from build123d import *

# Parameters (mm, degrees)
EXTRUDE1_DEPTH        = 3
SKETCH2_R             = 4
EXTRUDE2_DEPTH        = 9.5
SKETCH3_R             = 3
EXTRUDE3_DEPTH        = 11.5
SKETCH4_R             = 1.25
EXTRUDE4_DEPTH        = 10
SKETCH5_R             = 1.5
EXTRUDE5_DEPTH        = 3
M3_TAPPED_HOLE1_D     = 2.5
M3_TAPPED_HOLE1_DEPTH = 7.5
M3_TAPPED_HOLE1_TIP   = 0.751075774


with BuildPart() as part:
    # Sketch1 → Extrude1 (new body)
    with BuildSketch(Plane.XY):
        with BuildLine():
            Line((10, 4), (0, 4))
            ThreePointArc((0, 4), (-2.828427125, 2.828427125), (-4, 0))
            Line((-4, 0), (-4, -10))
            ThreePointArc((-4, -10), (5.899494937, -5.899494937), (10, 4))
        make_face()
    extrude(amount=EXTRUDE1_DEPTH)

    # Sketch2 → Extrude2 (add)
    with BuildSketch(Plane.XY.offset(3)):
        with Locations(Location((0, 0, 0), (0, 0, 180))):
            Circle(SKETCH2_R)
    extrude(amount=EXTRUDE2_DEPTH)

    # Sketch3 → Extrude3 (add)
    with BuildSketch(Plane.XY.offset(12.5)):
        Circle(SKETCH3_R)
    extrude(amount=EXTRUDE3_DEPTH)

    # Sketch4 → Extrude4 (cut)
    with BuildSketch(Plane.XY.offset(24)):
        Circle(SKETCH4_R)
    extrude(amount=-EXTRUDE4_DEPTH, mode=Mode.SUBTRACT)

    # Sketch5 → Extrude5 (cut)
    with BuildSketch(Plane.XY.offset(3)):
        with Locations((7, 1)):
            Circle(SKETCH5_R)
        with Locations((-1, -7)):
            Circle(SKETCH5_R)
    extrude(amount=-EXTRUDE5_DEPTH, mode=Mode.SUBTRACT)

    # M3 Tapped Hole1
    with Locations(Plane.XY.offset(24)):
        with Locations((0, 0)):
            Hole(M3_TAPPED_HOLE1_D / 2, depth=M3_TAPPED_HOLE1_DEPTH)
            with Locations((0, 0, -(M3_TAPPED_HOLE1_DEPTH + M3_TAPPED_HOLE1_TIP / 2))):  # 118° drill point
                Cone(0, M3_TAPPED_HOLE1_D / 2, M3_TAPPED_HOLE1_TIP, mode=Mode.SUBTRACT)


solid = part.part
Verification items for the finished model (mm, model axes). A direction names the side the tool comes from. Give positions to 0.01 mm unless a question says otherwise; leave off trailing zeros. Loops run counter-clockwise (first coordinate to the right, second up) from the corner with the lowest first, then second, coordinate; pieces in that order, holes last. Notation, with made-up numbers: (77.25, 28) - (114.25, 28) arc R37 cw to (114.25, 64) - close; hole circle Ø1 at (-39, 35.5). An arc over 180 degrees is marked (long way). Write item = value, one per line. Start each with the question number.
Q1. Mould release check, pull along Y, two halves, no side actions. Record for faces 3 (the face through (-0.27, -1.22, 19.07)), 4 (the face through (-1, -3, 12.5)), 5 (the face through (-1.325, -8.464, 1.521)), 6 (the face through (-3, 0, 18)): released by +Y, released by -Y, zero draft, split by the parting line, or undercut.
Q2. Depth check by flat-ended pin: P1, Ø5, axis at y = -5, z = 7.5, coming from the +X side; P2, Ø3, axis at y = 2, z = 10.5, coming from the -X side; P3, Ø3, axis at x = 5, y = 1.5, coming from the +Z side; P4, Ø2, axis at y = -4.5, z = 20.5, coming from the -X side. Enter the tip coordinate at first touch or a pass-through.
Q3. Tool access check on faces 1 (the face through (5.5, 1.07, 1.52)), 2 (the face through (0, 0, 14)). Record the directions out of +Z, -Z, +X, -X, +Y, -Y that give a thin tool (end or side, any length) a straight path to the whole face; none if there is none.
Q4. Cross-section at A-A, the plane y = 1. Enter the section's corners in (x, z).
Q5. Thickness scan on line 1 (Y direction, x = 0, z = 18.5); line 2 (Y direction, x = 7, z = 2.1); line 3 (Z direction, x = 1.5, y = -7.25). Record the ranges inside material, lowest first.
Q6. Cross-section at B-B, the plane x = -1. Enter the section's corners in (y, z).
Q7. Cross-section at C-C, the plane z = 22.25. Enter the section's corners in (x, y).
Q8. Cross-section at D-D, the plane x = 0.75. Enter the section's corners in (y, z), and give its area (3 significant figures).
Answer key:
q1.face_3 = undercut
q1.face_4 = zero draft
q1.face_5 = undercut
q1.face_6 = split by the parting line
q2.P1 = 3.12
q2.P2 = -3.97
q2.P3 = 12.5
q2.P4 = through
q3.face_1 = +Z, -Z
q3.face_2 = +Z
q4.outline = (-3.87, 0) - (5.5, 0) - (5.5, 3) - (3.87, 3) - (3.87, 12.5) - (2.83, 12.5) - (2.83, 24) - (0.75, 24) - (0.75, 14) - (-0.75, 14) - (-0.75, 24) - (-2.83, 24) - (-2.83, 12.5) - (-3.87, 12.5) - close; (8.5, 0) - (9.67, 0) - (9.67, 3) - (8.5, 3) - close
q5.line_1 = -3 to -1.25, 1.25 to 3
q5.line_2 = -4.66 to -0.5, 2.5 to 4
q5.line_3 = 0 to 3
q6.outline = (-9.67, 0) - (-8.5, 0) - (-8.5, 3) - (-9.67, 3) - close; (-5.5, 0) - (3.87, 0) - (3.87, 12.5) - (2.83, 12.5) - (2.83, 24) - (0.75, 24) - (0.75, 14) - (-0.75, 14) - (-0.75, 24) - (-2.83, 24) - (-2.83, 12.5) - (-3.87, 12.5) - (-3.87, 3) - (-5.5, 3) - close
q7.outline = circle Ø6 at (0, 0); hole circle Ø2.5 at (0, 0)
q8.outline = (-9.17, 0) - (4, 0) - (4, 3) - (3.93, 3) - (3.93, 12.5) - (2.9, 12.5) - (2.9, 24) - (1, 24) - (1, 14) - (-1, 14) - (-1, 24) - (-2.9, 24) - (-2.9, 12.5) - (-3.93, 12.5) - (-3.93, 3) - (-9.17, 3) - close
q8.area = 161 mm^2
